Here's the drawing with two shaded views (mm, measured from the low corner). I have some questions. Coordinates: 2 decimals unless noted, no trailing zeros. Loops run counter-clockwise (first coordinate to the right, second up) from the corner with the lowest first, then second, coordinate; pieces in that order, holes last. Notation, with made-up numbers: (80.5, 69) - (96.5, 69) arc R6 ccw to (96.5, 73) - close; hole circle Ø3 at (59.25, 37.25). An arc over 180 degrees is marked (long way). One line per item, written item: value. Start each with the question number.
(1) If we section it at C-C on z = 0.85: Write out the boundary of the cut face in (x, y), then the cut area to 3 significant figures.
(2) If I drill on line 1 along Y through (x, z) = (6, 1.05); line 2 along Y through (x, z) = (45, 0.4); line 3 along X through (y, z) = (3.75, 1.85), over which ranges is the centre line in solid material (lowest first)? Write a range as from..to.
(3) If we section it at B-B on y = 5: Write out the boundary of the cut face in (x, z), then the cut area to 3 significant figures.
(4) If we section it at D-D on x = 41: Write out the boundary of the cut face in (y, z).
(5) If we section it at A-A on x = 15: Write out the boundary of the cut face in (y, z).
(6) I'm going to push a flat-ended pin straight in: P1, Ø1.8, axis at x = 15, y = 5, coming from the +Z side. Where does the tip first touch, or does it pass through?
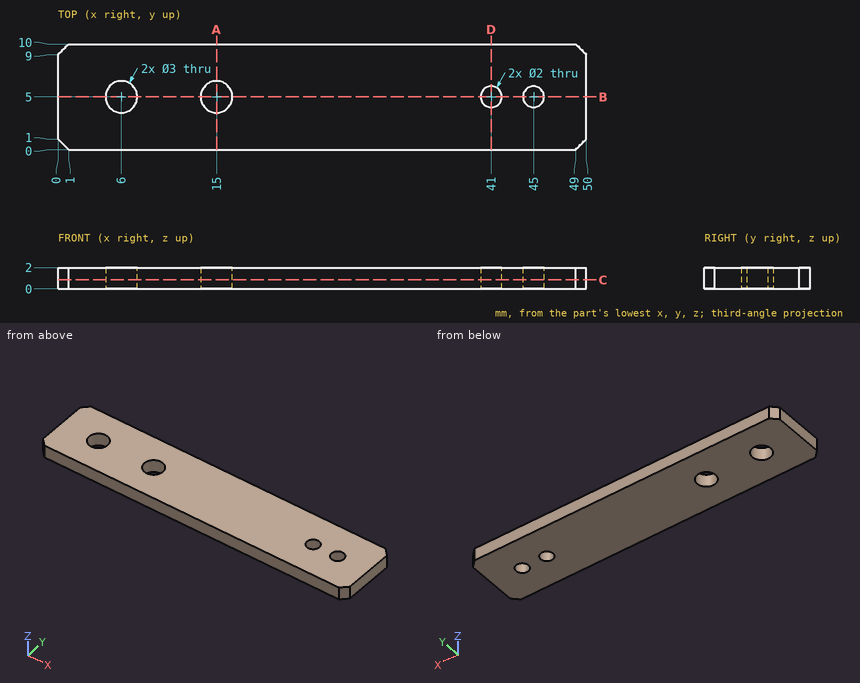
Values:
1. outline: (0, 1) - (1, 0) - (49, 0) - (50, 1) - (50, 9) - (49, 10) - (1, 10) - (0, 9) - close; hole circle Ø3 at (6, 5); hole circle Ø3 at (15, 5); hole circle Ø2 at (41, 5); hole circle Ø2 at (45, 5)
1. area: 478 mm2
2. line 1: y = 0..3.5, 6.5..10
2. line 2: y = 0..4, 6..10
2. line 3: x = 0..5.17, 6.83..14.17, 15.83..50
3. outline: (0, 0) - (4.5, 0) - (4.5, 2) - (0, 2) - close; (7.5, 0) - (13.5, 0) - (13.5, 2) - (7.5, 2) - close; (16.5, 0) - (40, 0) - (40, 2) - (16.5, 2) - close; (42, 0) - (44, 0) - (44, 2) - (42, 2) - close; (46, 0) - (50, 0) - (50, 2) - (46, 2) - close
3. area: 80.0 mm2
4. outline: (0, 0) - (4, 0) - (4, 2) - (0, 2) - close; (6, 0) - (10, 0) - (10, 2) - (6, 2) - close
5. outline: (0, 0) - (3.5, 0) - (3.5, 2) - (0, 2) - close; (6.5, 0) - (10, 0) - (10, 2) - (6.5, 2) - close
6. P1: passes through
